The figure shows three views and two pictorial views of one solid part (mm, origin at its lowest corner). Answer the questions. A direction names the side the tool comes from. Give positions to 0.01 mm unless a question says otherwise; leave off trailing zeros. Write each loop counter-clockwise with the first axis right and the second up, starting at its lowest first coordinate (ties: lowest second). Pieces come first, ordered by that corner, then holes. Notation, with made-up numbers: (23.5, 16) -> (46.5, 16) arc R26 cw to (46.5, 37) -> close; hole circle Ø6 at (46.5, 2.5). An arc over 180 degrees is marked (long way). Answer as CSV lines item,"result". Start each with the question number.
1. For a pull along Z with two mould halves and no side action, classify the marked faces 3, 4, 5 and 6 as pulls with the +Z half, pulls with the -Z half, needs draft (parallel to the pull), parting line crosses it, or undercut.
2. The part is cut by section D-D, the plane x = 50.5. Determine the outline of the cut face in (y, z).
3. A tool of negligible diameter and unlimited length cuts with its end or side. For the marked faces 1 and 2, from which of +Z, -Z, +X, -X, +Y, -Y can it reach the whole face along a straight path? Write none if from no direction.
4. The part is cut by section B-B, the plane z = 35. Determine the outline of the cut face in (x, y).
5. The part is cut by section A-A, the plane x = 30. Determine the outline of the cut face in (y, z), and give its area (3 significant figures).
6. The part is cut by section C-C, the plane y = 3.25. Determine the outline of the cut face in (x, z), and give its area (3 significant figures).
7. Find the intervals of material crossed by line 1 (Z direction, x = 30, y = 7.75); line 2 (Y direction, x = 25, z = 5); line 3 (Z direction, x = 38, y = 11.5), in increasing order.
8. Given pin 1 (8 mm diameter, centred on x = 22, y = 20.5, fed in from -Z); pin 2 (6 mm diameter, centred on y = 13, z = 47, fed in from +X); pin 3 (10 mm diameter, centred on y = 21, z = 10, fed in from -X), each flat-ended and moving along its own axis, determine where each tip first touches the part or whether it passes through.
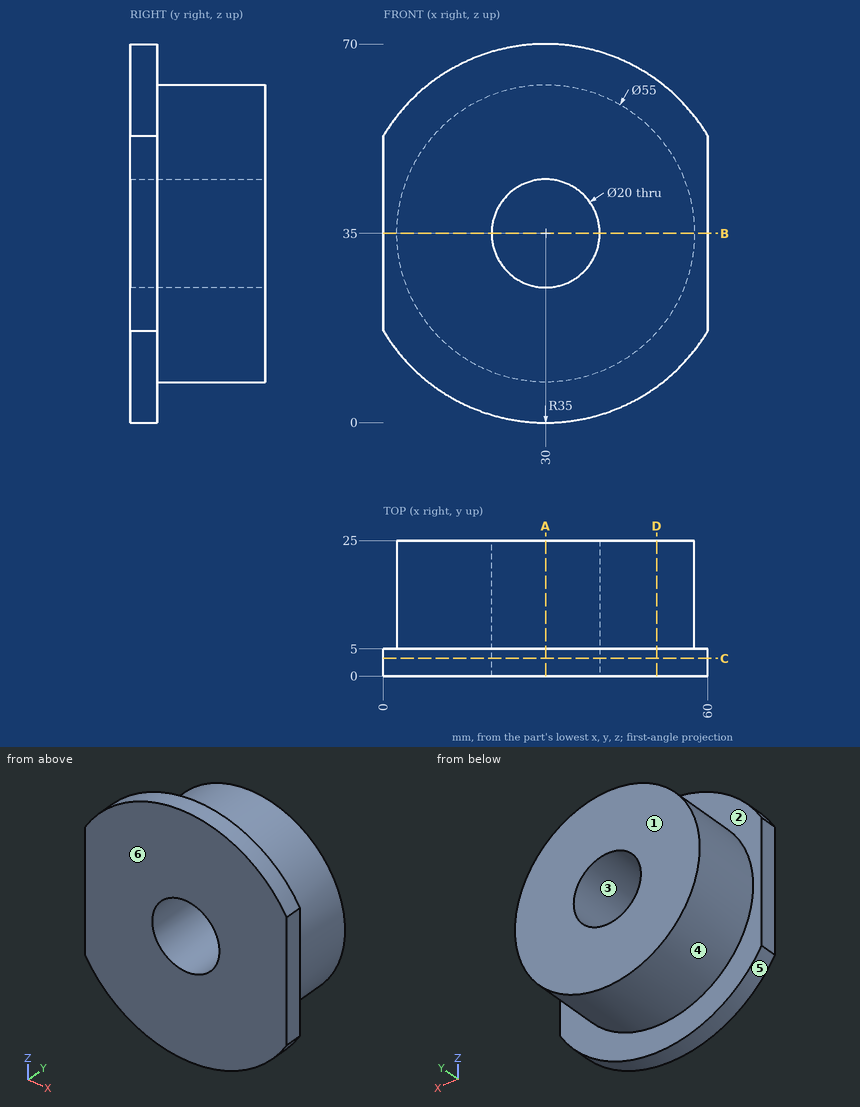
Results found:
1,face 3,"undercut"
1,face 4,"parting line crosses it"
1,face 5,"pulls with the -Z half"
1,face 6,"needs draft"
2,outline,"(0, 6.63) -> (5, 6.63) -> (5, 16.67) -> (25, 16.67) -> (25, 53.33) -> (5, 53.33) -> (5, 63.37) -> (0, 63.37) -> close"
3,face 1,"+Z, -Z, +X, -X, +Y"
3,face 2,"+Y"
4,outline,"(0, 0) -> (20, 0) -> (20, 25) -> (2.5, 25) -> (2.5, 5) -> (0, 5) -> close; (40, 0) -> (60, 0) -> (60, 5) -> (57.5, 5) -> (57.5, 25) -> (40, 25) -> close"
5,outline,"(0, 0) -> (5, 0) -> (5, 7.5) -> (25, 7.5) -> (25, 25) -> (0, 25) -> close; (0, 45) -> (25, 45) -> (25, 62.5) -> (5, 62.5) -> (5, 70) -> (0, 70) -> close"
5,area,"950 mm²"
6,outline,"(0, 16.97) arc R35 ccw to (60, 16.97) -> (60, 53.03) arc R35 ccw to (0, 53.03) -> close; hole circle Ø20 at (30, 35)"
6,area,"3,290 mm²"
7,line 1,"z = 7.5 to 25, 45 to 62.5"
7,line 2,"y = 0 to 5"
7,line 3,"z = 8.69 to 29, 41 to 61.31"
8,pin 1,"stops at z = 7.79"
8,pin 2,"stops at x = 55.99"
8,pin 3,"stops at x = 11.13"
